Can you work these out from the model? Positions are in its coordinate system, mm. A direction names the side the tool comes from. Round coordinates to 2 decimals unless told otherwise and drop trailing zeros. Loops run counter-clockwise (first coordinate to the right, second up) from the corner with the lowest first, then second, coordinate; pieces in that order, holes last.
from build123d import *

# Parameters (mm, degrees)
F0_R     = 5
F0_R_2   = 1.5
F1_DEPTH = 6
F0_R_3   = 3
F2_DEPTH = 4


with BuildPart() as f1:
    # F0 (on Top) → F1 (new body)
    with BuildSketch(Plane.XY):
        with BuildLine():
            ThreePointArc((-44.496753, -11.833806), (-46.710703, -14.496996), (-46.663059, -17.959925))
            ThreePointArc((-46.663059, -17.959925), (-43.30127, -25), (-38.885281, -31.431432))
            ThreePointArc((-38.885281, -31.431432), (-35.910118, -33.204157), (-32.496753, -32.618416))
            Line((-32.496753, -32.618416), (-15, -22.51666))
            ThreePointArc((-15, -22.51666), (0, -18.497423), (15, -22.51666))
            Line((15, -22.51666), (32.496753, -32.618416))
            ThreePointArc((32.496753, -32.618416), (35.910118, -33.204157), (38.885281, -31.431432))
            ThreePointArc((38.885281, -31.431432), (43.30127, -25), (46.663059, -17.959925))
            ThreePointArc((46.663059, -17.959925), (46.710703, -14.496996), (44.496753, -11.833806))
            Line((44.496753, -11.833806), (27, -1.732051))
            ThreePointArc((27, -1.732051), (16.019238, 9.248711), (12, 24.248711))
            Line((12, 24.248711), (12, 44.452222))
            ThreePointArc((12, 44.452222), (10.800585, 47.701153), (7.777778, 49.391357))
            ThreePointArc((7.777778, 49.391357), (0, 50), (-7.777778, 49.391357))
            ThreePointArc((-7.777778, 49.391357), (-10.800585, 47.701153), (-12, 44.452222))
            Line((-12, 44.452222), (-12, 24.248711))
            ThreePointArc((-12, 24.248711), (-16.019238, 9.248711), (-27, -1.732051))
            Line((-27, -1.732051), (-44.496753, -11.833806))
        make_face()
        with Locations((-30.310889, -17.5)):
            Circle(F0_R, mode=Mode.SUBTRACT)
        with Locations((-8.660254, -5)):
            Circle(F0_R_2, mode=Mode.SUBTRACT)
        with Locations((-8.660254, 5)):
            Circle(F0_R_2, mode=Mode.SUBTRACT)
        with Locations((30.310889, -17.5)):
            Circle(F0_R, mode=Mode.SUBTRACT)
        with Locations((0, -10)):
            Circle(F0_R_2, mode=Mode.SUBTRACT)
        with Locations((8.660254, -5)):
            Circle(F0_R_2, mode=Mode.SUBTRACT)
        Circle(F0_R, mode=Mode.SUBTRACT)
        with Locations((8.660254, 5)):
            Circle(F0_R_2, mode=Mode.SUBTRACT)
        with Locations((0, 10)):
            Circle(F0_R_2, mode=Mode.SUBTRACT)
        with Locations((0, 35)):
            Circle(F0_R, mode=Mode.SUBTRACT)
    extrude(amount=F1_DEPTH)

    # F0 (on Top) → F2 (join)
    with BuildSketch(Plane.XY):
        with Locations((-30.310889, -17.5)):
            Circle(F0_R)
        with Locations((-30.310889, -17.5)):
            Circle(F0_R_3, mode=Mode.SUBTRACT)
        with Locations((0, 35)):
            Circle(F0_R)
        with Locations((0, 35)):
            Circle(F0_R_3, mode=Mode.SUBTRACT)
        with Locations((30.310889, -17.5)):
            Circle(F0_R)
        with Locations((30.310889, -17.5)):
            Circle(F0_R_3, mode=Mode.SUBTRACT)
    extrude(amount=F2_DEPTH)


solid = f1.part
(1) If we section it at D-D, the plane y = 16.5: List the corners of the cut face in (x, z) for me, then the cut area to 3 significant figures.
Worked answers:
outline: (-13.02, 0) - (13.02, 0) - (13.02, 6) - (-13.02, 6) - close
area: 156 mm2
(2) If I drill on line 1 (Y direction, x = 0, z = 2.9); line 2 (X direction, y = 35.5, z = 4.35); line 3 (X direction, y = -22, z = 2.5), over which ranges is the centre line in solid material (lowest first)?
Worked answers:
line 1: y = -18.5 to -11.5, -8.5 to -5, 5 to 8.5, 11.5 to 32, 38 to 50
line 2: x = -12 to -4.97, 4.97 to 12
line 3: x = -44.9 to -14.07, 14.07 to 44.9
(3) Will these pins go through, and if not, where does the flat tip stop? P1, Ø7, axis at x = 30.31, y = -17.5, coming from the +Z side; P2, Ø3, axis at x = 33.5, y = -2, coming from the +Z side; P3, Ø1, axis at x = 35.5, z = 2.5, coming from the +Y side; P4, Ø1.8, axis at y = 39, z = 2.5, coming from the -X side.
Worked answers:
P1: stops at z = 4
P2: passes through
P3: stops at y = -6.35
P4: stops at x = -12
(4) For faces 1 (the cylindrical face through (26.34, -20.54, 4.99)), 2 (the flat face through (-12, 34, 3)), 3 (the cylindrical face through (-0.325, 8.536, 2.958)), which set-ups out of +Z, -Z, +X, -X, +Y, -Y let a thin tool reach every point of the face, with its end or its side?
Worked answers:
face 1: +Z
face 2: +Z, -Z, -X, +Y
face 3: +Z, -Z
(5) If we section it at C-C, the plane y = 0: List the corners of the cut face in (x, z) for me.
Worked answers:
outline: (-24.34, 0) - (-5, 0) - (-5, 6) - (-24.34, 6) - close; (5, 0) - (24.34, 0) - (24.34, 6) - (5, 6) - close
(6) If we section it at B-B, the plane y = 35: List the corners of the cut face in (x, z) for me, then the cut area to 3 significant figures.
Worked answers:
outline: (-12, 0) - (-3, 0) - (-3, 4) - (-5, 4) - (-5, 6) - (-12, 6) - close; (3, 0) - (12, 0) - (12, 6) - (5, 6) - (5, 4) - (3, 4) - close
area: 100 mm2
(7) If we section it at A-A, the plane x = 0: List the corners of the cut face in (y, z) for me, then the cut area to 3 significant figures.
Worked answers:
outline: (-18.5, 0) - (-11.5, 0) - (-11.5, 6) - (-18.5, 6) - close; (-8.5, 0) - (-5, 0) - (-5, 6) - (-8.5, 6) - close; (5, 0) - (8.5, 0) - (8.5, 6) - (5, 6) - close; (11.5, 0) - (32, 0) - (32, 4) - (30, 4) - (30, 6) - (11.5, 6) - close; (38, 0) - (50, 0) - (50, 6) - (40, 6) - (40, 4) - (38, 4) - close
area: 271 mm2
(8) If we mould it in two halves opening along Y, with no side actions, what happens to faces 4 (the flat face through (34, -17, 4)), 5 (the flat face through (12, 34, 3)), 6 (the flat face through (-23.87, -27.64, 2.96))? For each: released by +Y, released by -Y, zero draft, split by the parting line, or undercut.
Worked answers:
face 4: undercut
face 5: zero draft
face 6: released by -Y
